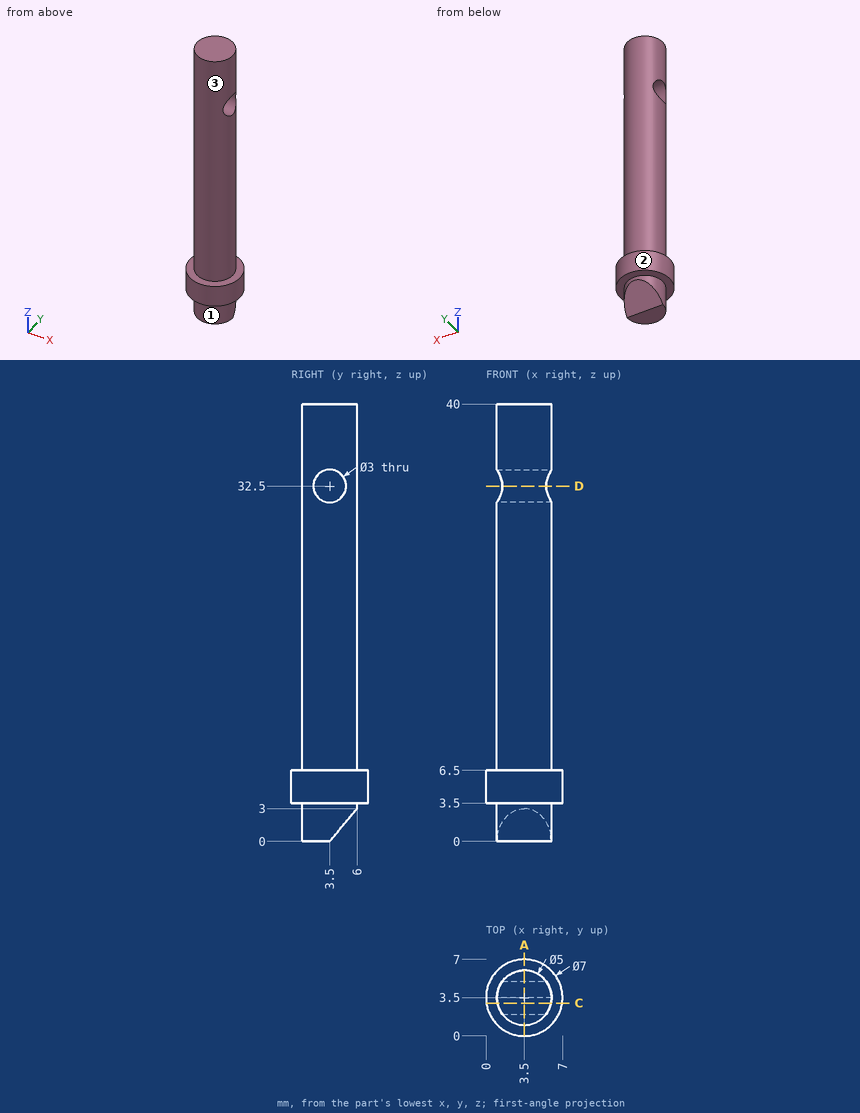
The drawing under review shows one solid part. Ordinate dimensions are in mm from its lowest x, y, z. A direction names the side the tool comes from. Give positions to 0.01 mm unless a question says otherwise; leave off trailing zeros. Order: outer loops, then holes, each group sorted by start corner. A loop starts at its lowest first (then second) coordinate and runs counter-clockwise, first axis right, second up. Notation, with made-up numbers: (85, 57.5) -> (124, 57.5) arc R22 ccw to (124, 95.5) -> close; hole circle Ø10 at (86, 23). An arc over 180 degrees is marked (long way). Write item = value, one per line.
1) We need section A-A, the plane x = 3.5. Give the boundary of the cut face in (y, z), and give its area (3 significant figures).
Findings:
outline = (0, 3.5) -> (1, 3.5) -> (1, 0) -> (3.5, 0) -> (6, 3) -> (6, 3.5) -> (7, 3.5) -> (7, 6.5) -> (6, 6.5) -> (6, 40) -> (1, 40) -> (1, 6.5) -> (0, 6.5) -> close; hole circle Ø3 at (3.5, 32.5)
area = 195 mm^2
2) Insertion check: pin 1 (2 mm diameter, centred on y = 5.5, z = 7, fed in from +X); pin 2 (1.8 mm diameter, centred on y = 3.5, z = 32.5, fed in from -X); pin 3 (1.5 mm diameter, centred on y = 4.5, z = 23.5, fed in from -X); pin 4 (1 mm diameter, centred on x = 1.5, y = 1, fed in from +Z). Each pin has a flat end and moves straight along its axis. Give the tip position at first contact, or say it passes through.
Findings:
pin_1 = 6.81
pin_2 = through
pin_3 = 1.01
pin_4 = 6.5
3) For the marked faces 1, 2 and 3, list the 3-axis set-ups (+Z, -Z, +X, -X, +Y, -Y) from which the entire face can be reached by the end or side of a thin tool; tool diameter is ignored.
Findings:
face_1 = -Z
face_2 = +Z, -Z
face_3 = +Z
4) To check wall thickness, follow L1, parallel to Y at x = 3.6, z = 32.5; L2, parallel to X at y = 3.5, z = 26; L3, parallel to Z at x = 3.5, y = 0.75. State the ranges of each line that lie inside material, in increasing order. Write a range as from..to.
Findings:
L1 = 1..2, 5..6
L2 = 1..6
L3 = 3.5..6.5
5) We need section C-C, the plane y = 3. Give the boundary of the cut face in (x, z).
Findings:
outline = (0.04, 3.5) -> (1.05, 3.5) -> (1.05, 0) -> (5.95, 0) -> (5.95, 3.5) -> (6.96, 3.5) -> (6.96, 6.5) -> (5.95, 6.5) -> (5.95, 31.09) -> (1.05, 31.09) -> (1.05, 6.5) -> (0.04, 6.5) -> close; (1.05, 33.91) -> (5.95, 33.91) -> (5.95, 40) -> (1.05, 40) -> close
6) We need section D-D, the plane z = 32.5. Give the boundary of the cut face in (x, y).
Findings:
outline = (1.5, 2) arc R2.5 ccw to (5.5, 2) -> close; (1.5, 5) -> (5.5, 5) arc R2.5 ccw to start
